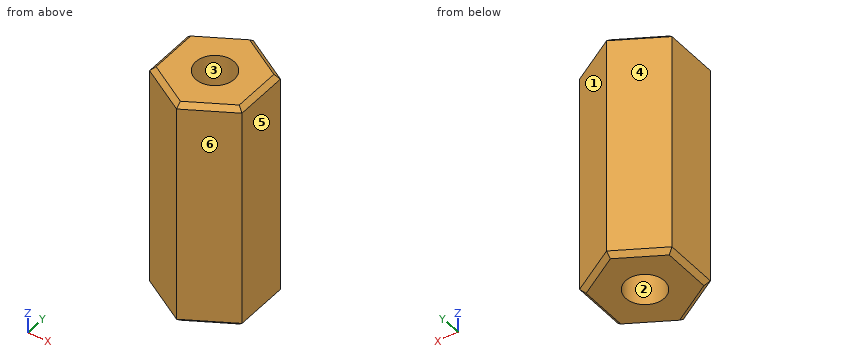
```python
from build123d import *

# Parameters (mm, degrees)
BOSS_EXTRUDE1_DEPTH   = 15
M3_TAPPED_HOLE1_D     = 2.5
M3_TAPPED_HOLE1_DEPTH = 6
M3_TAPPED_HOLE1_TIP   = 0.751075774
M3_TAPPED_HOLE2_D     = 2.5
M3_TAPPED_HOLE2_DEPTH = 7
M3_TAPPED_HOLE2_TIP   = 0.751075774
CHAMFER1_SIZE         = 0.3


with BuildPart() as part:
    # Sketch1 → Boss-Extrude1 (new body)
    with BuildSketch(Plane.XY):
        Polygon((0, 3.464101615), (-3, 1.732050808), (-3, -1.732050808), (0, -3.464101615), (3, -1.732050808), (3, 1.732050808), align=None)
    extrude(amount=BOSS_EXTRUDE1_DEPTH)

    # M3 Tapped Hole1
    with Locations(Plane.XY.offset(15)):
        with Locations((0, 0)):
            Hole(M3_TAPPED_HOLE1_D / 2, depth=M3_TAPPED_HOLE1_DEPTH)
            with Locations((0, 0, -(M3_TAPPED_HOLE1_DEPTH + M3_TAPPED_HOLE1_TIP / 2))):  # 118° drill point
                Cone(0, M3_TAPPED_HOLE1_D / 2, M3_TAPPED_HOLE1_TIP, mode=Mode.SUBTRACT)

    # M3 Tapped Hole2
    with Locations(Plane(origin=(0, 0, 0), x_dir=(-1, 0, 0), z_dir=(0, 0, -1))):
        with Locations((0, 0)):
            Hole(M3_TAPPED_HOLE2_D / 2, depth=M3_TAPPED_HOLE2_DEPTH)
            with Locations((0, 0, -(M3_TAPPED_HOLE2_DEPTH + M3_TAPPED_HOLE2_TIP / 2))):  # 118° drill point
                Cone(0, M3_TAPPED_HOLE2_D / 2, M3_TAPPED_HOLE2_TIP, mode=Mode.SUBTRACT)

    # Chamfer1
    chamfer1_edges = [part.edges().sort_by_distance(p)[0] for p in [
        (-3, 0, 15),
        (-1.5, -2.598076211, 15),
        (1.5, -2.598076211, 15),
        (3, 0, 15),
        (1.5, 2.598076211, 15),
        (3, 0, 0),
        (1.5, -2.598076211, 0),
        (-1.5, -2.598076211, 0),
        (-1.5, 2.598076211, 15),
        (-3, 0, 0),
        (-1.5, 2.598076211, 0),
        (1.5, 2.598076211, 0),
    ]]
    chamfer(chamfer1_edges, length=CHAMFER1_SIZE)


solid = part.part
```
Could you check a few things on this model? Use its own coordinates, in mm. Face numbers are marked on the shaded views. A direction names the side the tool comes from. Coordinates: 2 decimals unless noted, no trailing zeros. Write each loop counter-clockwise with the first axis right and the second up, starting at its lowest first coordinate (ties: lowest second). Pieces come first, ordered by that corner, then holes. Notation, with made-up numbers: (31, 15) -> (35, 15) arc R6 cw to (35, 24) -> close; hole circle Ø9 at (5.25, -12.5). An arc over 180 degrees is marked (long way). Return JSON: item names as keys, results as strings.
(1) Which directions (+Z, -Z, +X, -X, +Y, -Y) give clear straight access to the entire face, cutting with the end or side of a thin tool? Please do the marked faces 1 and 2.
Numbers:
{"face 1": "+Z, -Z, +X, +Y", "face 2": "-Z"}
(2) I'm going to push flat-ended pins straight in: pin 1 (1 mm diameter, centred on x = 1.5, z = 3.5, fed in from +Y); pin 2 (1.5 mm diameter, centred on x = 2, z = 13.5, fed in from -Y). Where does each tip first touch, or does it pass through?
Numbers:
{"pin 1": "stops at y = 2.89", "pin 2": "stops at y = -2.74"}
(3) Imagine slicing it at C-C, the plane z = 8. Please give me the cut outline in (x, y), then the cut area to 3 significant figures.
Numbers:
{"outline": "(-3, -1.73) -> (0, -3.46) -> (3, -1.73) -> (3, 1.73) -> (0, 3.46) -> (-3, 1.73) -> close", "area": "31.2 mm2"}
(4) I need wall thicknesses on L1, parallel to X at y = 0, z = 4; L2, parallel to Y at x = 0.25, z = 7.5; L3, parallel to Y at x = -0.75, z = 13.25. Which ranges of each line are inside material? Lowest first, please.
Numbers:
{"L1": "x = -3 to -1.25, 1.25 to 3", "L2": "y = -3.32 to -0.33, 0.33 to 3.32", "L3": "y = -3.03 to -1, 1 to 3.03"}
(5) Imagine slicing it at A-A, the plane z = 3.75. Please give me the cut outline in (x, y).
Numbers:
{"outline": "(-3, -1.73) -> (0, -3.46) -> (3, -1.73) -> (3, 1.73) -> (0, 3.46) -> (-3, 1.73) -> close; hole circle Ø2.5 at (0, 0)"}
(6) We'd pull the mould along Y, two halves only. Please class the marked faces 3, 4, 5 and 6: +Y half, -Y half, draft (parallel to the pull), parting line (faces both ways), or undercut.
Numbers:
{"face 3": "undercut", "face 4": "+Y half", "face 5": "draft", "face 6": "-Y half"}
(7) Imagine slicing it at B-B, the plane x = -1.5. Please give me the cut outline in (y, z).
Numbers:
{"outline": "(-2.6, 0.3) -> (-2.25, 0) -> (2.25, 0) -> (2.6, 0.3) -> (2.6, 14.7) -> (2.25, 15) -> (-2.25, 15) -> (-2.6, 14.7) -> close"}
(8) Imagine slicing it at D-D, the plane y = 2. Please give me the cut outline in (x, z).
Numbers:
{"outline": "(-2.54, 0.3) -> (-1.94, 0) -> (1.94, 0) -> (2.54, 0.3) -> (2.54, 14.7) -> (1.94, 15) -> (-1.94, 15) -> (-2.54, 14.7) -> close"}
